Geometry: final body of the model. Coordinates: model frame, mm. A direction names the side the tool comes from. Round coordinates to 2 decimals unless told otherwise and drop trailing zeros. Loops run counter-clockwise (first coordinate to the right, second up) from the corner with the lowest first, then second, coordinate; pieces in that order, holes last. Notation, with made-up numbers: M 21.25,-4 L 67.25,-4 A19 cw 67.25,32 Z; hole C 28,48 d5. An arc over 180 degrees is marked long. Write each question's results on one line, items separated by ' | '.
```python
from build123d import *

# Parameters (mm, degrees)
SKETCH1_R                   = 20.32
CYLINDER_DEPTH              = 14.478
SKETCH2_W                   = 7.62
SKETCH2_H                   = 11.938
SKETCH3_W                   = 2.286
SKETCH3_H                   = 2.794
SKETCH4_W                   = 8.87476
SKETCH4_H                   = 6.604
SKETCH5_W                   = 2.286
SKETCH5_H                   = 2.794
BOTTOM_CHAMFER_SIZE         = 3.81
BOTTOM_CHAMFER_SIZE2        = 1.27
MOUNTING_HOLE_REACH         = 34.178
SKETCH6_R                   = 1.27
MOUNTING_HOLE_PATTERN_COUNT = 6


with BuildPart() as part:
    # Sketch1 → Cylinder (new body)
    with BuildSketch(Plane(origin=(0, 0, 0), x_dir=(1, 0, 0), z_dir=(0, 1, 0))):
        with Locations(Location((0, 0, 0), (0, 0, 270))):
            Circle(SKETCH1_R)
    extrude(amount=CYLINDER_DEPTH)

    # Sketch2 → Mid O Ring Wings (revolve, cut)
    with BuildSketch(Plane.XY, mode=Mode.PRIVATE) as mid_o_ring_wings_sk:
        with Locations((16.51, 5.969)):
            Rectangle(SKETCH2_W, SKETCH2_H)
    revolve(mid_o_ring_wings_sk.sketch.rotate(Axis((0, 21.496286204, 0), (0, -1, 0)), 90), axis=Axis((0, 21.496286204, 0), (0, -1, 0)), mode=Mode.SUBTRACT)

    # Sketch3 → Mid O Ring Cut (revolve, cut)
    with BuildSketch(Plane.XY, mode=Mode.PRIVATE) as mid_o_ring_cut_sk:
        with Locations((11.557, 9.271)):
            Rectangle(SKETCH3_W, SKETCH3_H)
    revolve(mid_o_ring_cut_sk.sketch.rotate(Axis((0, 21.496286204, 0), (0, -1, 0)), 90), axis=Axis((0, 21.496286204, 0), (0, -1, 0)), mode=Mode.SUBTRACT)

    # Sketch4 → Bottom O Ring Wings (revolve, cut)
    with BuildSketch(Plane.XY, mode=Mode.PRIVATE) as bottom_o_ring_wings_sk:
        with Locations((8.26262, 3.302)):
            Rectangle(SKETCH4_W, SKETCH4_H)
    revolve(bottom_o_ring_wings_sk.sketch.rotate(Axis((0, 21.496286204, 0), (0, -1, 0)), 90), axis=Axis((0, 21.496286204, 0), (0, -1, 0)), mode=Mode.SUBTRACT)

    # Sketch5 → Bottom O Ring Cut (revolve, cut)
    with BuildSketch(Plane.XY, mode=Mode.PRIVATE) as bottom_o_ring_cut_sk:
        with Locations((2.68224, 3.937)):
            Rectangle(SKETCH5_W, SKETCH5_H)
    revolve(bottom_o_ring_cut_sk.sketch.rotate(Axis((0, 21.496286204, 0), (0, -1, 0)), 90), axis=Axis((0, 21.496286204, 0), (0, -1, 0)), mode=Mode.SUBTRACT)

    # Bottom Chamfer
    bottom_chamfer_edges = [part.edges().sort_by_distance(p)[0] for p in [
        (0, 0, -3.82524),
    ]]
    bottom_chamfer_side = [part.faces().sort_by_distance(p)[0] for p in [
        (0, 0, 0),
    ]]
    chamfer(bottom_chamfer_edges, length=BOTTOM_CHAMFER_SIZE, length2=BOTTOM_CHAMFER_SIZE2, reference=bottom_chamfer_side[0])

    # Sketch6 → Mounting Hole (cut, up to next)
    with BuildSketch(Plane(origin=(0, 14.478, 0), x_dir=(1, 0, 0), z_dir=(0, 1, 0)), mode=Mode.PRIVATE) as mounting_hole_sk1:
        with Locations(Location((0, 17.78, 0), (0, 0, 270))):
            Circle(SKETCH6_R)
    mounting_hole_tool1 = extrude(mounting_hole_sk1.sketch, amount=-MOUNTING_HOLE_REACH, mode=Mode.PRIVATE) & part.part
    mounting_hole = mounting_hole_tool1.solids().sort_by_distance((0, 14.478, -17.78))[0]
    add(mounting_hole, mode=Mode.SUBTRACT)

    # Mounting Hole Pattern: Mounting Hole ×6 about axis
    mounting_hole_pattern_axis = Axis((0, 0, 0), (0, 1, 0))
    for i in range(1, MOUNTING_HOLE_PATTERN_COUNT):
        add(mounting_hole.rotate(mounting_hole_pattern_axis, i * 360 / MOUNTING_HOLE_PATTERN_COUNT), mode=Mode.SUBTRACT)


solid = part.part
```
1. Ray query, probe 1 along Y at (x, z) = (-11.5, -3); probe 2 along X at (y, z) = (13.9, -8.89); probe 3 along Y at (x, z) = (-5, -7). Return the intervals inside material, ascending.
Answer key:
probe 1: y = 6.6 to 7.87, 10.67 to 14.48 | probe 2: x = -18.27 to -16.67, -14.13 to 14.13, 16.67 to 18.27 | probe 3: y = 6.6 to 14.48
2. Pin query (flat end, axial travel): P1, Ø3, axis at x = -15.4, z = -8.89, coming from the -Y side; P2, Ø1, axis at x = 12.5, y = 8.5, coming from the +Z side; P3, Ø4, axis at y = 10.5, z = 16, coming from the -X side; P4, Ø7.5, axis at x = -1.5, z = 3.5, coming from the -Y side. Return the tip coordinate at first contact, or that it passes through.
Answer key:
P1: stops at y = 11.94 | P2: passes through | P3: stops at x = -14.12 | P4: stops at y = 0.01
3. Section A-A (z = -17.78). Output: boundary loops of the cut face in (x, y), then the cut area to 3 significant figures.
Answer key:
outline: M -9.84,11.94 L -1.27,11.94 L -1.27,14.48 L -9.84,14.48 Z; M 1.27,11.94 L 9.84,11.94 L 9.84,14.48 L 1.27,14.48 Z | area: 43.5 mm²
4. Section B-B (x = -11). Output: boundary loops of the cut face in (y, z).
Answer key:
outline: M 6.6,-6.35 L 7.87,-6.35 L 7.87,6.35 L 6.6,6.35 Z; M 10.67,-6.35 L 11.94,-6.35 L 11.94,-17.09 L 14.48,-17.09 L 14.48,17.09 L 11.94,17.09 L 11.94,6.35 L 10.67,6.35 Z
5. Access query for faces 1 (the face through (0.06, 13.23, -19.05)), 2 (the face through (-10.4, 7.874, 1.9)), 3 (the face through (-3, 6.604, -3)). Directions: +Z, -Z, +X, -X, +Y, -Y. A direction counts if a zero-diameter tool reaches every point of the face in a straight line with its end or side. Return the directions, or none.
Answer key:
face 1: +Y, -Y | face 2: none | face 3: -Y
6. Section C-C (z = -8.89). Output: boundary loops of the cut face in (x, y), then the cut area to 3 significant figures.
Answer key:
outline: M -18.27,11.94 L -16.67,11.94 L -16.67,14.48 L -18.27,14.48 Z; M -14.13,11.94 L -9.07,11.94 L -9.07,10.67 L -5.42,10.67 L -5.42,7.87 L -9.07,7.87 L -9.07,6.6 L 9.07,6.6 L 9.07,7.87 L 5.42,7.87 L 5.42,10.67 L 9.07,10.67 L 9.07,11.94 L 14.13,11.94 L 14.13,14.48 L -14.13,14.48 Z; M 16.67,11.94 L 18.27,11.94 L 18.27,14.48 L 16.67,14.48 Z | area: 156 mm²
7. Draft query along X for faces 4 (the face through (-14.54, 13.226, 7.954)), 5 (the face through (-0.46, 3.96, 1.47)), 6 (the face through (-10.4, 10.668, 1.9)). Return one class per face: pulls with the +X half, pulls with the -X half, needs draft (parallel to the pull), parting line crosses it, or undercut.
Answer key:
face 4: undercut | face 5: parting line crosses it | face 6: needs draft
8. Section D-D (x = -15.5). Output: boundary loops of the cut face in (y, z).
Answer key:
outline: M 11.94,-13.14 L 14.48,-13.14 L 14.48,-10.16 L 11.94,-10.16 Z; M 11.94,-7.62 L 14.48,-7.62 L 14.48,7.62 L 11.94,7.62 Z; M 11.94,10.16 L 14.48,10.16 L 14.48,13.14 L 11.94,13.14 Z
